```python
from build123d import *

# Parameters (mm, degrees)
F0_W      = 96
F0_H      = 28
F1_DEPTH  = 36
F2_W      = 20
F2_H      = 96
F3_DEPTH  = 20
F4_R      = 5
F5_R      = 4
F6_DEPTH  = 36
F7_R      = 6
F8_DEPTH  = 4
F9_SIZE   = 1
F10_R     = 3
F11_DEPTH = 8


with BuildPart() as f1:
    # F0 (on Right) → F1 (new body)
    with BuildSketch(Plane.YZ):
        with Locations((10.8510512412, -14)):
            Rectangle(F0_W, F0_H)
    extrude(amount=F1_DEPTH)

    # F2 (on face) → F3 (cut)
    with BuildSketch(Plane.XY):
        with Locations((18, 10.8510512412)):
            Rectangle(F2_W, F2_H)
    extrude(amount=-F3_DEPTH, mode=Mode.SUBTRACT)

    # F4
    f4_edges = [f1.edges().sort_by_distance(p)[0] for p in [
        (36, 10.851051, -28),
        (0, 10.851051, -28),
    ]]
    fillet(f4_edges, radius=F4_R)

    # F5 (on face) → F6 (cut)
    with BuildSketch(Plane.YZ.offset(36)):
        with Locations((46.8510512412, -10)):
            Circle(F5_R)
        with Locations((22.8510512412, -10)):
            Circle(F5_R)
        with Locations((-1.1489487588, -10)):
            Circle(F5_R)
        with Locations((-25.1489487588, -10)):
            Circle(F5_R)
    extrude(amount=-F6_DEPTH, mode=Mode.SUBTRACT)

    # F7 (on face) → F8 (cut)
    with BuildSketch(Plane.YZ.offset(36)):
        with Locations((-25.1489487588, -10)):
            Circle(F7_R)
        with Locations((-1.1489487588, -10)):
            Circle(F7_R)
        with Locations((22.8510512412, -10)):
            Circle(F7_R)
        with Locations((46.8510512412, -10)):
            Circle(F7_R)
    extrude(amount=-F8_DEPTH, mode=Mode.SUBTRACT)

    # F9
    f9_edges = [f1.edges().sort_by_distance(p)[0] for p in [
        (32, -29.148949, -10),
        (32, -5.148949, -10),
        (32, 18.851051, -10),
        (32, 42.851051, -10),
    ]]
    chamfer(f9_edges, length=F9_SIZE)

    # F10 (on face) → F11 (cut)
    with BuildSketch(Plane(origin=(0, 0, -28), x_dir=(1, 0, 0), z_dir=(0, 0, -1))):
        with Locations((18, -46.8510512412)):
            Circle(F10_R)
        with Locations((18, -10.8510512412)):
            Circle(F10_R)
        with Locations((18, 25.1489487588)):
            Circle(F10_R)
    extrude(amount=-F11_DEPTH, mode=Mode.SUBTRACT)


solid = f1.part
```
Work out the finished part from the listing and answer in its coordinate system (mm). A direction names the side the tool comes from. Give positions to 0.01 mm unless a question says otherwise; leave off trailing zeros. Loops run counter-clockwise (first coordinate to the right, second up) from the corner with the lowest first, then second, coordinate; pieces in that order, holes last. Notation, with made-up numbers: M 82,10.5 L 114,10.5 A3 ccw 114,14.5 Z; hole C 2.5,74.25 d7. An arc over 180 degrees is marked long. One line per item, written item: value. Start each with the question number.
1. Find section B-B (z = -17.5). Give the vertices of the cut face in (x, y), and give its area (3 significant figures).
2. Find section D-D (y = 32.5). Give the vertices of the cut face in (x, z).
3. Find section A-A (x = 29). Give the vertices of the cut face in (y, z).
4. Which of the six approach directions +Z, -Z, +X, -X, +Y, -Y give full straight-line access (tool end or side, diameter ignored) to faces 1 (the face through (34.03, -1.93, -4.05)), 2 (the face through (29.521, 26.546, -11.532))?
5. Find the intervals of material crossed by probe 1 along Y at (x, z) = (18, -23.5); probe 2 along Y at (x, z) = (28.5, -9.75); probe 3 along X at (y, z) = (-1, -16.25), in increasing order.
6. Each of these flat-tipped pins is pushed along its axis until it touches: P1, Ø6, axis at y = -25.5, z = -8.5, coming from the +X side; P2, Ø6, axis at x = 17, y = 35, coming from the +Z side; P3, Ø11, axis at y = -25.15, z = -10, coming from the +X side. Where does it stop, or does it pass through?
7. Find section C-C (x = 18). Give the vertices of the cut face in (y, z), and give its area (3 significant figures).
8. Determine the mould class of faces 3 (the face through (15.62, 12.68, -24.06)), 4 (the face through (17.7, 58.851, -20.4)), 5 (the face through (32, -3, -5)) for opening direction X: released by +X, released by -X, zero draft, split by the parting line, or undercut.
Reported:
1. outline: M 0,-37.15 L 8,-37.15 L 8,58.85 L 0,58.85 Z; M 28,-37.15 L 36,-37.15 L 36,58.85 L 28,58.85 Z
1. area: 1,540 mm²
2. outline: M 0,-23 A5 ccw 5,-28 L 31,-28 A5 ccw 36,-23 L 36,0 L 28,0 L 28,-20 L 8,-20 L 8,0 L 0,0 Z
3. outline: M -37.15,-28 L 58.85,-28 L 58.85,0 L -37.15,0 Z; hole C -25.15,-10 d8; hole C -1.15,-10 d8; hole C 22.85,-10 d8; hole C 46.85,-10 d8
4. face 1: +X
4. face 2: +X, -X
5. probe 1: y = -37.15 to -28.15, -22.15 to 7.85, 13.85 to 43.85, 49.85 to 58.85
5. probe 2: y = -37.15 to -29.14, -21.16 to -5.14, 2.84 to 18.86, 26.84 to 42.86, 50.84 to 58.85
5. probe 3: x = 0 to 8, 28 to 36
6. P1: stops at x = 31.54
6. P2: stops at z = -20
6. P3: stops at x = 32
7. outline: M -37.15,-28 L -28.15,-28 L -28.15,-20 L -37.15,-20 Z; M -22.15,-28 L 7.85,-28 L 7.85,-20 L -22.15,-20 Z; M 13.85,-28 L 43.85,-28 L 43.85,-20 L 13.85,-20 Z; M 49.85,-28 L 58.85,-28 L 58.85,-20 L 49.85,-20 Z
7. area: 624 mm²
8. face 3: undercut
8. face 4: zero draft
8. face 5: released by +X
